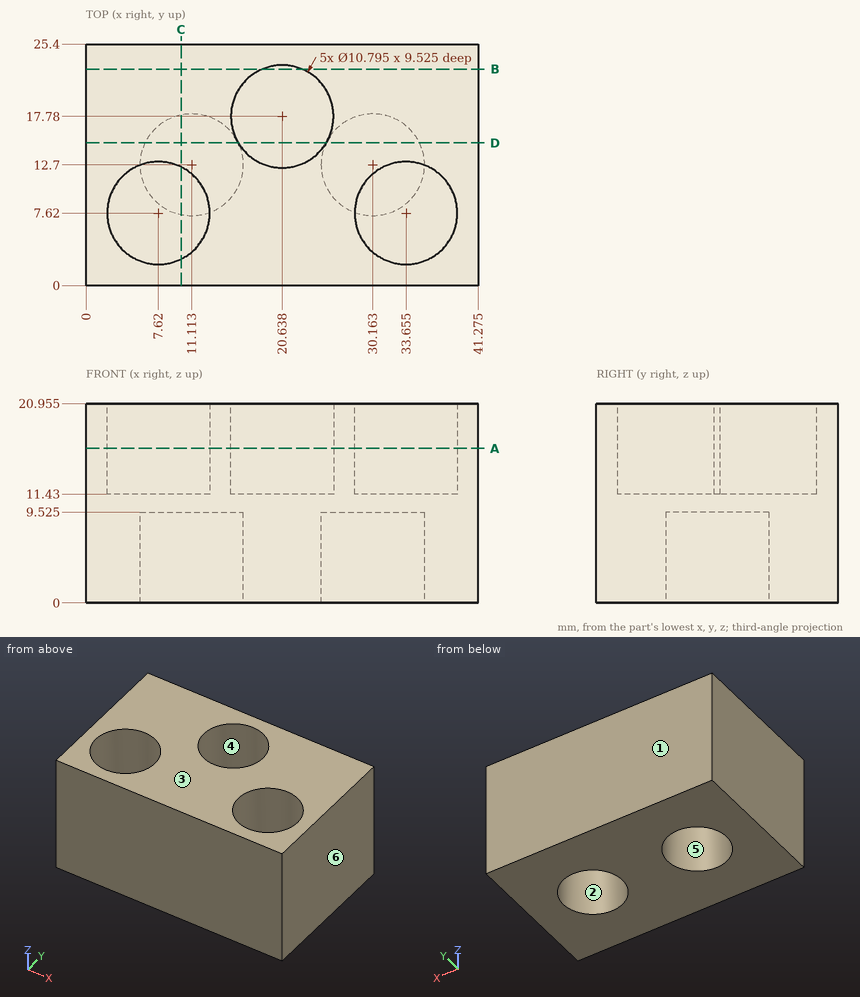
Drawing for the job (mm, zero at the part's lowest x, y, z). A direction names the side the tool comes from. Give positions to 0.01 mm unless a question says otherwise; leave off trailing zeros. Loops run counter-clockwise (first coordinate to the right, second up) from the corner with the lowest first, then second, coordinate; pieces in that order, holes last. Notation, with made-up numbers: M 46.5,89.25 L 81.5,89.25 A19 cw 81.5,126.25 Z; hole C -12,27 d4. An arc over 180 degrees is marked long. One line per question, with ' | ' between items. Start each with the question number.
1. 3-axis set-ups, long thin cutter, end or side, ignore diameter. For the marked faces 4, 5 and 6: which of +Z, -Z, +X, -X, +Y, -Y reach the whole face in a straight line?
2. Saw through at D-D on y = 15. Give the cut face in (x, z) (1 decimal), plus the area to 3 significant figures.
3. Two-plate mould, pull along Y, no slides. Class the marked faces 1, 2 and 3: pulls with the +Y half, pulls with the -Y half, needs draft (parallel to the pull), parting line crosses it, or undercut.
4. Probe L1, parallel to Y at x = 7.62, z = 16; L2, parallel to X at y = 9.5, z = 16.75 (1 decimal); L3, parallel to X at y = 16.75, z = 7 (1 decimal). List the from-to ranges inside material, lowest first. Write a range as from..to.
5. Flat gauge pins, fed straight in: pin 1 (3 mm diameter, centred on x = 14.5, y = 12.5, fed in from -Z) (1 decimal); pin 2 (5.5 mm diameter, centred on x = 20.5, y = 19.5, fed in from +Z). Where does each tip first touch, or does it go through?
6. Saw through at A-A on z = 16.25. Give the cut face in (x, y) (1 decimal).
7. Saw through at B-B on y = 22.75. Give the cut face in (x, z) (1 decimal), plus the area to 3 significant figures.
8. Saw through at C-C on x = 10. Give the cut face in (y, z) (1 decimal).
Result sheet:
1) face 4: +Z | face 5: -Z | face 6: +Z, -Z, +X, +Y, -Y
2) outline: M 0,0 L 6.2,0 L 6.2,9.5 L 16,9.5 L 16,0 L 25.3,0 L 25.3,9.5 L 35,9.5 L 35,0 L 41.3,0 L 41.3,21 L 25.3,21 L 25.3,11.4 L 16,11.4 L 16,21 L 0,21 Z | area: 591 mm^2
3) face 1: pulls with the +Y half | face 2: undercut | face 3: needs draft
4) L1: y = 0..2.22, 13.02..25.4 | L2: x = 0..2.6, 12.7..28.6, 38.7..41.3 | L3: x = 0..7.5, 14.7..26.6, 33.7..41.3
5) pin 1: stops at z = 9.5 | pin 2: stops at z = 11.43
6) outline: M 0,0 L 41.3,0 L 41.3,25.4 L 0,25.4 Z; hole C 7.6,7.6 d10.8; hole C 20.6,17.8 d10.8; hole C 33.7,7.6 d10.8
7) outline: M 0,0 L 41.3,0 L 41.3,21 L 22.7,21 L 22.7,11.4 L 18.5,11.4 L 18.5,21 L 0,21 Z | area: 825 mm^2
8) outline: M 0,0 L 7.4,0 L 7.4,9.5 L 18,9.5 L 18,0 L 25.4,0 L 25.4,21 L 12.5,21 L 12.5,11.4 L 2.8,11.4 L 2.8,21 L 0,21 Z
